Part model, mm, in its own coordinate system. Face numbers are marked on the shaded views. A direction names the side the tool comes from. Coordinates: 2 decimals unless noted, no trailing zeros. Order: outer loops, then holes, each group sorted by start corner. A loop starts at its lowest first (then second) coordinate and runs counter-clockwise, first axis right, second up.
1) Wall check: L1, parallel to Z at x = 8, y = 2.5; L2, parallel to Y at x = -18, z = 12; L3, parallel to Z at x = -22.5, y = 4.75. Give the ranges that are in metal, low to high.
2) Cut at A-A (x = -9). List the corners of the cut face in (y, z), and give its area (3 significant figures).
3) Cut at C-C (y = 2.75). List the corners of the cut face in (x, z), and give its area (3 significant figures).
4) Tool access for the marked faces 1, 2 and 3: list every direction of +Z, -Z, +X, -X, +Y, -Y with a clear straight run to the whole face (end or side of a thin tool).
5) Cut at B-B (z = -29.5). List the corners of the cut face in (x, y).
6) Mould opens along Y. For the marked faces 4, 5 and 6 say: +Y half, -Y half, draft (parallel to the pull), parting line (faces both ways), or undercut.
7) Pin check, flat tips, straight feed: pin 1 Ø3 at (x, z) = (-1.5, 12.5) entering from -Y; pin 2 Ø1.6 at (y, z) = (8.5, -10) entering from -X; pin 3 Ø2 at (y, z) = (5, -6.5) entering from +X; pin 4 Ø3 at (y, z) = (4, 18.5) entering from -X. Stop position of each tip, or through.
8) Cut at D-D (z = -8). List the corners of the cut face in (x, y), and give its area (3 significant figures).
Autodesk Inventor part; units mm, degrees
ref_plane "YZ Plane" through (0, 0, 0) normal (1, 0, 0) x (0, 1, 0)
ref_plane "XZ Plane" through (0, 0, 0) normal (0, 1, 0) x (-1, 0, 0)
ref_plane "XY Plane" through (0, 0, 0) normal (0, 0, 1) x (1, 0, 0)
sketch "Esquisse1" plane through (0, 0, 0) normal (0, 1, 0) x (-1, 0, 0)
  line L0 (-27.5, 32.5) -> (27.5, 32.5)
  line L1 (27.5, 32.5) -> (27.5, -32.5)
  line L2 (27.5, -32.5) -> (-27.5, -32.5)
  line L3 (-27.5, -32.5) -> (-27.5, 32.5)
  line L4 (-27.5, 32.5) -> (27.5, -32.5) construction
  line L5 (27.5, 32.5) -> (-27.5, -32.5) construction
  line L6 (-24.9615, 29.5) -> (24.9615, 29.5) construction
  line L7 (24.9615, 29.5) -> (24.9615, -29.5) construction
  line L8 (24.9615, -29.5) -> (-24.9615, -29.5) construction
  line L9 (-24.9615, -29.5) -> (-24.9615, 29.5) construction
  line L10 (-24.9615, 29.5) -> (24.9615, -29.5) construction
  line L11 (24.9615, 29.5) -> (-24.9615, -29.5) construction
  circle A0 centre (24.9615, 29.5) radius 1.65
  circle A1 centre (-24.9615, 29.5) radius 1.65
  circle A2 centre (-24.9615, -29.5) radius 1.65
  circle A3 centre (24.9615, -29.5) radius 1.65
  point P0 (0, 0)
  dimension "d0" = 65
  dimension "d1" = 55
  dimension "d3" = 3.3
  dimension "d6" = 3
extrude "Extrusion1" add sketch "Esquisse1" along normal blind 1.6
sketch "Esquisse2" plane through (0, 1.6, 0) normal (0, 1, 0) x (1, 0, 0)
  circle A0 centre (-24.9615, 29.5) radius 1.65 construction
  circle A1 centre (24.9615, 29.5) radius 1.65 construction
  circle A2 centre (24.9615, -29.5) radius 1.65 construction
  circle A3 centre (-24.9615, -29.5) radius 1.65 construction
  line L0 (-27.5, -32.5) -> (27.5, -32.5) construction
  line L1 (27.5, -32.5) -> (27.5, 32.5) construction
  line L2 (27.5, 32.5) -> (-27.5, 32.5) construction
  line L3 (-27.5, 32.5) -> (-27.5, -32.5) construction
  line L4 (-23.3115, -19.7912) -> (23.3115, -19.7912)
  line L5 (23.3115, -19.7912) -> (23.3115, -17.3453)
  line L6 (23.3115, -17.3453) -> (-23.3115, -17.3453)
  line L7 (-23.3115, -17.3453) -> (-23.3115, -19.7912)
  line L8 (-23.3115, -7.7912) -> (23.3115, -7.7912)
  line L9 (23.3115, -7.7912) -> (23.3115, -5.3453)
  line L10 (23.3115, -5.3453) -> (-23.3115, -5.3453)
  line L11 (-23.3115, -5.3453) -> (-23.3115, -7.7912)
  line L12 (-17.887, 0) -> (-15.6042, 0)
  line L13 (-15.6042, 0) -> (-15.6042, 17.3864)
  line L14 (-15.6042, 17.3864) -> (-17.887, 17.3864)
  line L15 (-17.887, 17.3864) -> (-17.887, 0)
  line L16 (0, 0) -> (19.7798, 0)
  line L17 (19.7798, 0) -> (19.7798, 2.0588)
  line L18 (19.7798, 2.0588) -> (0, 2.0588)
  line L19 (0, 2.0588) -> (0, 0)
  line L20 (0, 17) -> (19.7798, 17)
  line L21 (19.7798, 17) -> (19.7798, 19.0588)
  line L22 (19.7798, 19.0588) -> (0, 19.0588)
  line L23 (0, 19.0588) -> (0, 17)
  dimension "d9" = 12
  dimension "d16" = 17
extrude "Extrusion2" add sketch "Esquisse2" along normal blind 6
sketch "Esquisse3" plane through (0, 7.6, 0) normal (0, 1, 0) x (1, 0, 0)
  line L0 (-23.3115, -7.7912) -> (23.3115, -7.7912) construction
  line L1 (23.3115, -7.7912) -> (23.3115, -5.3453) construction
  line L2 (23.3115, -5.3453) -> (-23.3115, -5.3453) construction
  line L3 (-23.3115, -5.3453) -> (-23.3115, -7.7912) construction
  line L4 (-23.3115, -19.7912) -> (23.3115, -19.7912) construction
  line L5 (23.3115, -19.7912) -> (23.3115, -17.3453) construction
  line L6 (23.3115, -17.3453) -> (-23.3115, -17.3453) construction
  line L7 (-23.3115, -17.3453) -> (-23.3115, -19.7912) construction
  line L8 (0, 0) -> (19.7798, 0) construction
  line L9 (19.7798, 0) -> (19.7798, 2.0588) construction
  line L10 (19.7798, 2.0588) -> (0, 2.0588) construction
  line L11 (0, 2.0588) -> (0, 0) construction
  line L12 (0, 17) -> (19.7798, 17) construction
  line L13 (19.7798, 17) -> (19.7798, 19.0588) construction
  line L14 (19.7798, 19.0588) -> (0, 19.0588) construction
  line L15 (0, 19.0588) -> (0, 17) construction
  line L16 (-17.887, 0) -> (-15.6042, 0)
  line L17 (-15.6042, 0) -> (-15.6042, 17.3864)
  line L18 (-15.6042, 17.3864) -> (-17.887, 17.3864)
  line L19 (-17.887, 17.3864) -> (-17.887, 0)
  line L20 (-23.3115, -19.7912) -> (23.3115, -19.7912)
  line L21 (23.3115, -19.7912) -> (23.3115, -5.3453)
  line L22 (23.3115, -5.3453) -> (-23.3115, -5.3453)
  line L23 (-23.3115, -5.3453) -> (-23.3115, -19.7912)
  line L24 (19.7798, -1.6873) -> (19.7798, 20.7873)
  line L25 (19.7798, 20.7873) -> (1.1914, 20.7873)
  line L26 (1.1914, 20.7873) -> (-2.6949, 16.9011)
  line L27 (-2.6949, 16.9011) -> (-2.6949, 2.1989)
  line L28 (-2.6949, 2.1989) -> (1.1914, -1.6873)
  line L29 (1.1914, -1.6873) -> (19.7798, -1.6873)
  line L30 (1.1914, 20.7873) -> (1.1914, -1.6873) construction
  line L31 (-17.887, 0) -> (-5.5241, 0)
  line L32 (-5.5241, 0) -> (-5.5241, 17.3864)
  line L33 (-5.5241, 17.3864) -> (-17.887, 17.3864)
  line L34 (-17.887, 17.3864) -> (-17.887, 0)
extrude "Extrusion3" add sketch "Esquisse3" along normal blind 1.5
properties part number "board"
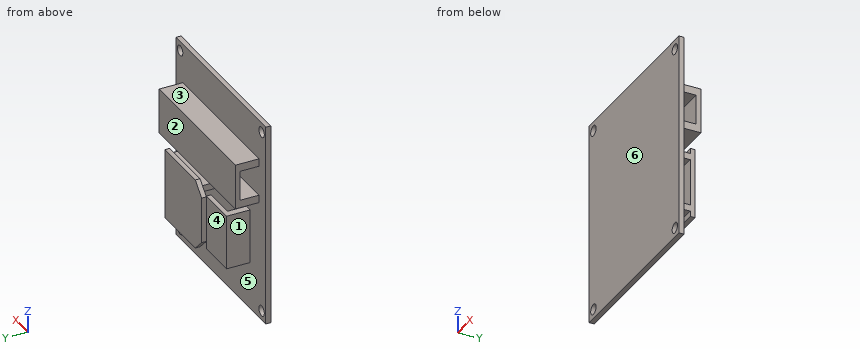
Geometry check:
1. L1: z = -19.06 to -17, -2.06 to 0, 5.35 to 7.79, 17.35 to 19.79
1. L2: y = 0 to 1.6, 7.6 to 9.1
1. L3: z = 5.35 to 7.79, 17.35 to 19.79
2. outline: (0, -32.5) - (1.6, -32.5) - (1.6, 5.35) - (9.1, 5.35) - (9.1, 19.79) - (1.6, 19.79) - (1.6, 32.5) - (0, 32.5) - close; (7.6, -17.39) - (9.1, -17.39) - (9.1, 0) - (7.6, 0) - close; hole (1.6, 7.79) - (7.6, 7.79) - (7.6, 17.35) - (1.6, 17.35) - close
2. area: 181 mm2
3. outline: (-23.31, 5.35) - (23.31, 5.35) - (23.31, 7.79) - (-23.31, 7.79) - close; (-23.31, 17.35) - (23.31, 17.35) - (23.31, 19.79) - (-23.31, 19.79) - close; (-17.89, -17.39) - (-15.6, -17.39) - (-15.6, 0) - (-17.89, 0) - close; (0, -19.06) - (19.78, -19.06) - (19.78, -17) - (0, -17) - close; (0, -2.06) - (19.78, -2.06) - (19.78, 0) - (0, 0) - close
3. area: 349 mm2
4. face 1: -Z, -X, +Y
4. face 2: +Z, -Z, +X, -X, +Y
4. face 3: +Z, +X, -X, +Y
5. outline: (-27.5, 0) - (-26.61, 0) - (-26.61, 1.6) - (-27.5, 1.6) - close; (-23.31, 0) - (23.31, 0) - (23.31, 1.6) - (-23.31, 1.6) - close; (26.61, 0) - (27.5, 0) - (27.5, 1.6) - (26.61, 1.6) - close
6. face 4: +Y half
6. face 5: undercut
6. face 6: -Y half
7. pin 1: stops at y = 0
7. pin 2: stops at x = -17.89
7. pin 3: stops at x = -15.6
7. pin 4: stops at x = -23.31
8. outline: (-27.5, 0) - (27.5, 0) - (27.5, 1.6) - (-15.6, 1.6) - (-15.6, 7.6) - (-5.52, 7.6) - (-5.52, 9.1) - (-17.89, 9.1) - (-17.89, 1.6) - (-27.5, 1.6) - close; (-2.69, 7.6) - (19.78, 7.6) - (19.78, 9.1) - (-2.69, 9.1) - close
8. area: 154 mm2
